from build123d import *

# Parameters (mm, degrees)
BOSS_EXTRUDE1_DEPTH            = 3
SKETCH2_W                      = 10
SKETCH2_H                      = 4.5
BOSS_EXTRUDE2_DEPTH            = 5
CUT_EXTRUDE1_DEPTH             = 2
F_2_2_2_2_DIAMETER_HOLE1_D     = 2.2
F_2_2_2_2_DIAMETER_HOLE1_DEPTH = 6.000025
F_6_2_6_2_DIAMETER_HOLE1_D     = 6.2
F_6_2_6_2_DIAMETER_HOLE1_DEPTH = 3
F_2_2_2_2_DIAMETER_HOLE2_D     = 2.2
F_2_2_2_2_DIAMETER_HOLE2_DEPTH = 3
F_2_5_2_5_DIAMETER_HOLE1_D     = 2.5
F_2_5_2_5_DIAMETER_HOLE1_DEPTH = 21.5
F_1_6_1_6_DIAMETER_HOLE1_D     = 1.6
F_1_6_1_6_DIAMETER_HOLE1_DEPTH = 4
F_1_6_1_6_DIAMETER_HOLE1_TIP   = 0.480688495
FILLET1_R                      = 2


with BuildPart() as part:
    # Sketch1 → Boss-Extrude1 (new body)
    with BuildSketch(Plane(origin=(0, 3, 0), x_dir=(1, 0, 0), z_dir=(0, 1, 0))):
        with BuildLine():
            Line((5.000000003, -5.193376137), (5.000000003, 0))
            Line((5.000000003, 0), (-4.999999997, 0))
            Line((-4.999999997, 0), (-4.999999997, -5.193376137))
            ThreePointArc((-4.999999997, -5.193376137), (-7.227019257, -9.084119567), (-7.999999997, -13.5))
            ThreePointArc((-7.999999997, -13.5), (3e-09, -21.5), (8.000000003, -13.5))
            ThreePointArc((8.000000003, -13.5), (7.227019264, -9.084119567), (5.000000003, -5.193376137))
        make_face()
    extrude(amount=-BOSS_EXTRUDE1_DEPTH)

    # Sketch2 → Boss-Extrude2 (add)
    with BuildSketch(Plane.XZ):
        with Locations((0, 2.25)):
            Rectangle(SKETCH2_W, SKETCH2_H)
    extrude(amount=BOSS_EXTRUDE2_DEPTH)

    # Sketch3 → Cut-Extrude1 (cut)
    with BuildSketch(Plane(origin=(0, 3, 0), x_dir=(-1, 0, 0), z_dir=(0, 1, 0))):
        with BuildLine():
            ThreePointArc((-2.053172912, 18.058999999), (-3.535533906, 17.035533905), (-4.559, 15.55317291))
            ThreePointArc((-4.559, 15.55317291), (-7.1, 13.5), (-4.559, 11.44682709))
            ThreePointArc((-4.559, 11.44682709), (-3.535533906, 9.964466094), (-2.053172911, 8.941))
            ThreePointArc((-2.053172911, 8.941), (0, 6.4), (2.05317291, 8.941))
            ThreePointArc((2.05317291, 8.941), (3.535533906, 9.964466094), (4.559, 11.44682709))
            ThreePointArc((4.559, 11.44682709), (7.1, 13.5), (4.559, 15.55317291))
            ThreePointArc((4.559, 15.55317291), (3.535533906, 17.035533906), (2.05317291, 18.059))
            ThreePointArc((2.05317291, 18.059), (-1e-09, 20.6), (-2.053172912, 18.058999999))
        make_face()
    extrude(amount=-CUT_EXTRUDE1_DEPTH, mode=Mode.SUBTRACT)

    # Ø2.2 (2.2) Diameter Hole1
    with Locations(Plane(origin=(0, 1, 0), x_dir=(1, 0, 0), z_dir=(0, 1, 0))):
        with Locations((-5, -13.5)):
            Hole(F_2_2_2_2_DIAMETER_HOLE1_D / 2, depth=F_2_2_2_2_DIAMETER_HOLE1_DEPTH)

    # Ø6.2 (6.2) Diameter Hole1
    with Locations(Plane(origin=(0, 0, 0), x_dir=(-1, 0, 0), z_dir=(0, -1, 0))):
        with Locations((0, -13.5)):
            Hole(F_6_2_6_2_DIAMETER_HOLE1_D / 2, depth=F_6_2_6_2_DIAMETER_HOLE1_DEPTH)

    # Ø2.2 (2.2) Diameter Hole2
    with Locations(Plane(origin=(0, 0, 0), x_dir=(-1, 0, 0), z_dir=(0, -1, 0))):
        with Locations((0, -8.5), (-5, -13.5), (0, -18.5)):
            Hole(F_2_2_2_2_DIAMETER_HOLE2_D / 2, depth=F_2_2_2_2_DIAMETER_HOLE2_DEPTH)

    # Ø2.5 (2.5) Diameter Hole1
    with Locations(Plane(origin=(0, 0, 0), x_dir=(-1, 0, 0), z_dir=(0, 0, -1))):
        with Locations((-1.5, -2)):
            Hole(F_2_5_2_5_DIAMETER_HOLE1_D / 2, depth=F_2_5_2_5_DIAMETER_HOLE1_DEPTH)

    # Ø1.6 (1.6) Diameter Hole1
    with Locations(Plane(origin=(0, 0, 0), x_dir=(-1, 0, 0), z_dir=(0, 0, -1))):
        with Locations((3, 1)):
            Hole(F_1_6_1_6_DIAMETER_HOLE1_D / 2, depth=F_1_6_1_6_DIAMETER_HOLE1_DEPTH)
            with Locations((0, 0, -(F_1_6_1_6_DIAMETER_HOLE1_DEPTH + F_1_6_1_6_DIAMETER_HOLE1_TIP / 2))):  # 118° drill point
                Cone(0, F_1_6_1_6_DIAMETER_HOLE1_D / 2, F_1_6_1_6_DIAMETER_HOLE1_TIP, mode=Mode.SUBTRACT)

    # Fillet1
    fillet1_edges = [part.edges().sort_by_distance(p)[0] for p in [
        (5.000000003, 1.5, 5.193376137),
        (-4.999999997, 1.5, 5.193376137),
    ]]
    fillet(fillet1_edges, radius=FILLET1_R)


solid = part.part
For this review, take the finished solid that the model builds, in its own axes (mm). A direction names the side the tool comes from. Give positions to 0.01 mm unless a question says otherwise; leave off trailing zeros. Order: outer loops, then holes, each group sorted by start corner. A loop starts at its lowest first (then second) coordinate and runs counter-clockwise, first axis right, second up. Notation, with made-up numbers: (42.25, 68) -> (69.25, 68) arc R18 cw to (69.25, 97) -> close; hole circle Ø9 at (39.25, 50). An arc over 180 degrees is marked (long way). Write item = value, one per line.
1) Insertion check: pin 1 (2 mm diameter, centred on x = 1.5, y = -2, fed in from -Z); pin 2 (2.5 mm diameter, centred on x = 5, z = 13.5, fed in from -Y); pin 3 (1.5 mm diameter, centred on y = -1, z = 4, fed in from -X); pin 4 (4 mm diameter, centred on x = 0, z = 18.5, fed in from +Y). Each pin has a flat end and moves straight along its axis. Give the tip position at first contact, or say it passes through.
Findings:
pin_1 = through
pin_2 = 0
pin_3 = -5
pin_4 = 1
2) We need section B-B, the plane z = 8.5. Give the boundary of the cut face in (x, y).
Findings:
outline = (-7, 0) -> (-1.1, 0) -> (-1.1, 1) -> (-2.1, 1) -> (-2.1, 3) -> (-7, 3) -> close; (1.1, 0) -> (7, 0) -> (7, 3) -> (2.1, 3) -> (2.1, 1) -> (1.1, 1) -> close
3) For faces 1 (the face through (7.1, 2.01, 13.55)), 2 (the face through (-3.7, 0, 12.9)), 3 (the face through (5, -1, 2)), list the 3-axis set-ups (+Z, -Z, +X, -X, +Y, -Y) from which the entire face can be reached by the end or side of a thin tool; tool diameter is ignored.
Findings:
face_1 = +Y
face_2 = +Z, +X, -X, -Y
face_3 = -Z, +X, +Y, -Y
4) We need section A-A, the plane y = -2. Give the boundary of the cut face in (x, z), and give its area (4 significant figures).
Findings:
outline = (-5, 0) -> (0.25, 0) -> (0.25, 4.5) -> (-5, 4.5) -> close; (2.75, 0) -> (5, 0) -> (5, 4.5) -> (2.75, 4.5) -> close
area = 33.75 mm^2
5) To check wall thickness, follow L1, parallel to X at y = 0.5, z = 13.5; L2, parallel to Z at x = 0, y = 2.1; L3, parallel to Y at x = -1.5, z = 19. State the ranges of each line that lie inside material, in increasing order. Write a range as from..to.
Findings:
L1 = -8..-6.1, -3.9..-3.1, 3.1..3.9, 6.1..8
L2 = 0..6.4, 20.6..21.5
L3 = 0..1
6) Draft analysis for pull direction X (two halves, no side actions). For faces 4 (the face through (5.117, 1.352, 5.175)), 5 (the face through (-2.237, 1.24, 2.028)), 6 (the face through (-5.1, 1.48, 5.12)), state which applies: pulls with the +X half, pulls with the -X half, needs draft (parallel to the pull), parting line crosses it, or undercut.
Findings:
face_4 = pulls with the +X half
face_5 = undercut
face_6 = pulls with the -X half
7) We need section D-D, the plane x = 0. Give the boundary of the cut face in (y, z).
Findings:
outline = (-5, 0) -> (3, 0) -> (3, 6.4) -> (1, 6.4) -> (1, 7.4) -> (0, 7.4) -> (0, 4.5) -> (-5, 4.5) -> close; (0, 9.6) -> (1, 9.6) -> (1, 10.4) -> (0, 10.4) -> close; (0, 16.6) -> (1, 16.6) -> (1, 17.4) -> (0, 17.4) -> close; (0, 19.6) -> (1, 19.6) -> (1, 20.6) -> (3, 20.6) -> (3, 21.5) -> (0, 21.5) -> close
8) We need section C-C, the plane x = -1.75. Give the boundary of the cut face in (y, z).
Findings:
outline = (-5, 0) -> (3, 0) -> (3, 7.34) -> (1, 7.34) -> (1, 10.94) -> (0, 10.94) -> (0, 4.5) -> (-5, 4.5) -> close; (0, 16.06) -> (1, 16.06) -> (1, 19.66) -> (3, 19.66) -> (3, 21.31) -> (0, 21.31) -> close
